```python
from build123d import *

# Parameters (mm, degrees)
F2_DEPTH = 20
F4_R     = 1.625
F7_DEPTH = 3
F8_R     = 1.25
F9_DEPTH = 2.4010001
F10_R    = 3
F11_R    = 1


with BuildPart() as f2:
    # F1 (on Front) → F2 (new body)
    with BuildSketch(Plane.XZ):
        with BuildLine():
            Line((18, 0), (0, 0))
            Line((0, 0), (-18, 0))
            Line((-18, 0), (-18, -2.4))
            Line((-18, -2.4), (-8, -2.4))
            ThreePointArc((-8, -2.4), (0, -10.4), (8, -2.4))
            Line((8, -2.4), (18, -2.4))
            Line((18, -2.4), (18, 0))
        make_face()
    extrude(amount=F2_DEPTH)

    # F5: sweep along a path in F3
    with BuildLine(Plane.YZ) as f5_path:
        Line((0, -3), (-5.1303021499, -3))
        ThreePointArc((-5.1303021499, -3), (-7.7350248149, -3.2278837048), (-10.2606042998, -3.9046106882))
        Line((-10.2606042998, -3.9046106882), (-24.8597601286, -9.2182688553))
    # F4 (on face) → F5 (sweep, cut)
    with BuildSketch(Plane(origin=(0, 0, 0), x_dir=(-1, 0, 0), z_dir=(0, 1, 0))):
        with Locations((0, -3)):
            Circle(F4_R)
    sweep(path=f5_path.line, mode=Mode.SUBTRACT)

    # F6 (on face) → F7 (cut)
    with BuildSketch(Plane.XY):
        Polygon((1.625, -9.5), (1.625, -5.1303021499), (1.625, 0), (-1.625, 0), (-1.625, -5.1303021499), (-1.625, -9.5), align=None)
    extrude(amount=-F7_DEPTH, mode=Mode.SUBTRACT)

    # F8 (on face) → F9 (cut, through all)
    with BuildSketch(Plane(origin=(0, 0, -2.4), x_dir=(1, 0, 0), z_dir=(0, 0, -1))):
        with Locations((13, 13.3333333333)):
            Circle(F8_R)
        with Locations((13, 6.6666666667)):
            Circle(F8_R)
        with Locations((-13, 13.3333333333)):
            Circle(F8_R)
        with Locations((-13, 6.6666666667)):
            Circle(F8_R)
    extrude(amount=-F9_DEPTH, mode=Mode.SUBTRACT)

    # F10
    f10_edges = [f2.edges().sort_by_distance(p)[0] for p in [
        (18, -20, -1.2),
        (18, 0, -1.2),
        (-18, -20, -1.2),
        (-18, 0, -1.2),
    ]]
    fillet(f10_edges, radius=F10_R)

    # F11
    f11_edges = [f2.edges().sort_by_distance(p)[0] for p in [
        (0, -20, -10.4),
        (-11.5, -20, -2.4),
        (11.5, -20, -2.4),
        (0, 0, -10.4),
    ]]
    fillet(f11_edges, radius=F11_R)


solid = f2.part
```
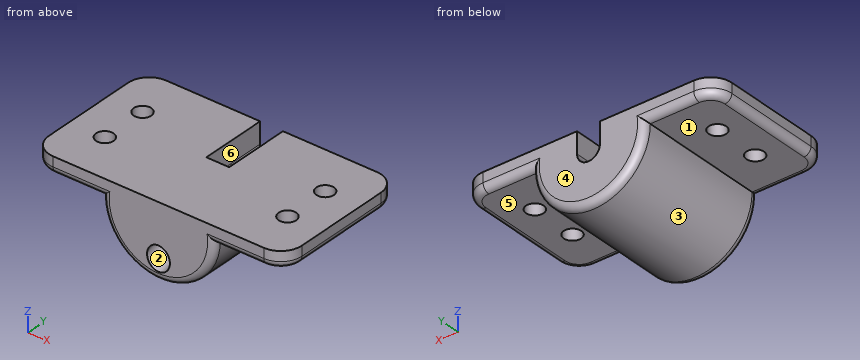
Read the model definition and answer for the solid it produces. Units are mm, in the model's axes. Face numbers are marked on the shaded views. A direction names the side the tool comes from. Round coordinates to 2 decimals unless told otherwise and drop trailing zeros. Loops run counter-clockwise (first coordinate to the right, second up) from the corner with the lowest first, then second, coordinate; pieces in that order, holes last. Notation, with made-up numbers: (63.5, 75.5) -> (82.5, 75.5) arc R23 cw to (82.5, 106.5) -> close; hole circle Ø5 at (76, 76). An arc over 180 degrees is marked (long way). One line per item, written item: value.
1) Consider L1, parallel to Y at x = -13, z = -0.6; L2, parallel to Z at x = 12, y = -1.25; L3, parallel to X at y = -2.5, z = -0.5 (3 decimals). Determine where each line is inside the solid, lowest interval first. Write a range as [from, to].
Answer list:
L1: y = [-20, -14.58], [-12.08, -7.92], [-5.42, 0]
L2: z = [-2.4, 0]
L3: x = [-17.958, -1.625], [1.625, 17.958]
2) Flat-ended cylindrical pins translate along their axes: P1, Ø8, axis at x = -9.5, y = -6.5, coming from the +Z side; P2, Ø1, axis at x = 7.5, z = -6, coming from the +Y side; P3, Ø5, axis at y = -3, z = -4, coming from the -X side (3 decimals); P4, Ø2.5, axis at x = -10.5, y = -9, coming from the -Z side. Find the tip coordinate at first contact, or state that the pin passes through.
Answer list:
P1: stops at z = 0
P2: stops at y = -0.43
P3: stops at x = -17.995
P4: stops at z = -2.4
3) A cutting plane is placed at A-A (x = 13). Determine the outline of the cut face in (y, z), and give its area (3 significant figures).
Answer list:
outline: (-20, -1.4) arc R1 ccw to (-19, -2.4) -> (-14.58, -2.4) -> (-14.58, 0) -> (-20, 0) -> close; (-12.08, -2.4) -> (-7.92, -2.4) -> (-7.92, 0) -> (-12.08, 0) -> close; (-5.42, -2.4) -> (-1, -2.4) arc R1 ccw to (0, -1.4) -> (0, 0) -> (-5.42, 0) -> close
area: 35.6 mm²
4) A cutting plane is placed at B-B (y = -4.75). Determine the outline of the cut face in (x, z) (3 decimals), and give its area (3 significant figures).
Answer list:
outline: (-18, -1.4) arc R1 ccw to (-17, -2.4) -> (-8, -2.4) arc R8 ccw to (8, -2.4) -> (17, -2.4) arc R1 ccw to (18, -1.4) -> (18, 0) -> (1.625, 0) -> (1.625, -3) arc R1.625 cw to (-1.625, -3) -> (-1.625, 0) -> (-18, 0) -> close
area: 173 mm²
5) A cutting plane is placed at D-D (x = 8.5). Determine the outline of the cut face in (y, z).
Answer list:
outline: (-20, -1.4) arc R1 ccw to (-19, -2.4) -> (-1, -2.4) arc R1 ccw to (0, -1.4) -> (0, 0) -> (-20, 0) -> close
6) The mould has two halves that part along X. Classify the marked faces 1, 2 and 3: pulls with the +X half, pulls with the -X half, needs draft (parallel to the pull), parting line crosses it, or undercut.
Answer list:
face 1: needs draft
face 2: undercut
face 3: parting line crosses it
7) A cutting plane is placed at C-C (x = 0). Determine the outline of the cut face in (y, z) (3 decimals), and give its area (3 significant figures).
Answer list:
outline: (-20, -9.4) arc R1 ccw to (-19, -10.4) -> (-1, -10.4) arc R1 ccw to (0, -9.4) -> (0, -4.625) -> (-5.13, -4.625) arc R13.375 ccw to (-9.705, -5.432) -> (-20, -9.179) -> close; (-20, -5.72) -> (-10.816, -2.378) arc R16.625 cw to (-9.5, -1.96) -> (-9.5, 0) -> (-20, 0) -> close
area: 126 mm²
8) For the marked faces 4, 5 and 6, determine the directions among +Z, -Z, +X, -X, +Y, -Y from which every point of the face is accessible in a straight line to the end or side of a thin tool.
Answer list:
face 4: +Z, -Z, +X, -X, +Y
face 5: -Z, +X, +Y, -Y
face 6: +Z, +Y
